The listing builds one solid part. Answer for the finished solid, in the listing's coordinates (mm). A direction names the side the tool comes from. Coordinates: 2 decimals unless noted, no trailing zeros. Write each loop counter-clockwise with the first axis right and the second up, starting at its lowest first coordinate (ties: lowest second). Pieces come first, ordered by that corner, then holes. Notation, with made-up numbers: M -21.5,36 L 12.5,36 A17 cw 12.5,46 Z; hole C 44,43.25 d1. An arc over 180 degrees is marked long. Answer as a JSON object with one key per item and string values. Group by question number.
Autodesk Inventor part; units mm, degrees
ref_plane "YZ Plane" through (0, 0, 0) normal (1, 0, 0) x (0, 1, 0)
ref_plane "XZ Plane" through (0, 0, 0) normal (0, 1, 0) x (-1, 0, 0)
ref_plane "XY Plane" through (0, 0, 0) normal (0, 0, 1) x (1, 0, 0)
sketch "Sketch1" plane through (0, 0, 0) normal (0, 0, 1) x (1, 0, 0)
  circle A0 centre (0, 0) radius 60.5
  circle A1 centre (0, 0) radius 55
  line L0 (0, 55) -> (-10, 55)
  line L1 (0, 55) -> (10, 55)
  line L2 (0, 55) -> (10, 55) construction
  line L3 (10, 59.6678) -> (10, 53.8845)
  line L4 (-10, 59.6678) -> (-10, 54.0833)
  point P0 (10, 54.0833)
  dimension "d0" = 121
  dimension "d1" = 110
  dimension "d45" = 10
  dimension "d46" = 10
  dimension "d47" = 0
extrude "Extrusion1" add sketch "Sketch1" along normal blind 2
extrude "Extrusion2" add sketch "Sketch1" against normal blind 8 contours A0 L4 A1 L3 | L3 L1 L0 L4 A0 | L3 A1 L1 | L0 A1 L4
sketch "Sketch11" plane through (0, 0, 0) normal (1, 0, 0) x (0, 1, 0)
  line L0 (60.5, 2) -> (-60.5, 2)
  line L1 (-60.5, -8) -> (60.5, -8)
  line L2 (59.6678, 0) -> (54.0833, 0)
  line L3 (59.6678, 0) -> (59.6678, -6)
  line L4 (54.0833, -6) -> (59.6678, -6)
  line L5 (54.0833, 0) -> (54.0833, -6)
  line L6 (-60.5, -8) -> (60.5, -8)
  line L7 (55, -8) -> (-55, -8)
  line L8 (-60.5, -8) -> (60.5, -8)
  line L9 (60.5, 0) -> (-60.5, 0)
  line L10 (-55, -8) -> (-61, -8)
  line L11 (-61, -8) -> (-61, 0)
  line L12 (-61, 0) -> (-55, 0)
  line L13 (-55, 0) -> (-55, -8)
  line L14 (-61, -8) -> (-55, 0)
  circle A0 centre (-58, -4) radius 2.1
  line L15 (-61, -8) -> (-67, -8)
  line L16 (-67, -8) -> (-67, -2)
  line L17 (-67, -2) -> (-61, -2)
  line L18 (-61, -2) -> (-61, -8)
  line L19 (-61, -8) -> (-67, -2)
  circle A1 centre (-64, -5) radius 2.15
  point P0 (0, 0)
  point P1 (42.0833, 0)
  point P2 (42.0833, -6)
  point P3 (48.0833, -6)
  dimension "d48" = 6
  dimension "d49" = 4.2
  dimension "d50" = 6
  dimension "d51" = 6
  dimension "d52" = 4.3
sketch "Sketch12" plane through (0, 0, 2) normal (0, 0, 1) x (1, 0, 0)
  point P0 (0, 0)
sketch "Sketch13" plane through (0, 0, 0) normal (0, 1, 0) x (-1, 0, 0)
  line L0 (0, -6) -> (0, 2)
  line L1 (0, 0) -> (0, -1)
  line L2 (0, -1) -> (3.1, -1)
  line L3 (3.1, -1) -> (3.1, -7.2)
  line L4 (3.1, -7.2) -> (0, -7.2)
  line L5 (0, -7.2) -> (0, -1)
  line L6 (3.1, -7.2) -> (-3.1, -7.2)
  line L7 (-3.1, -7.2) -> (-3.1, -1)
  line L8 (-3.1, -1) -> (3.1, -1)
  line L9 (3.1, -1) -> (3.1, -7.2)
  line L10 (0, -4.1) -> (6, -4.1)
  line L11 (6, -4.1) -> (-6, -4.1)
  circle A0 centre (-6, -4.1) radius 2.15
  circle A1 centre (6, -4.1) radius 2.15
  point P0 (0, -7.2)
  dimension "d58" = 1
  dimension "d59" = 3.1
  dimension "d60" = 6.2
  dimension "d61" = 6.2
  dimension "d62" = 6.2
  dimension "d66" = 6
  dimension "d67" = 12
  dimension "d68" = 4.3
  dimension "d69" = 4.3
extrude "Extrusion12" cut sketch "Sketch13" along normal through all
fillet "Fillet3" radius 0.3 4 edges at (-3.1, 57.6665, -1) (3.1, 57.6665, -1) (3.1, 57.6665, -7.2) (-3.1, 57.6665, -7.2)
sketch "Sketch14" plane through (0, 0, -8) normal (0, 0, -1) x (-1, 0, 0)
  circle A0 centre (0, 0) radius 57.5
  circle A1 centre (0, 57.5) radius 2.4
  circle A2 centre (-49.7965, -28.75) radius 2.4
  circle A3 centre (49.7965, -28.75) radius 2.4
  point P0 (50.9528, -26.6469)
  point P1 (48.5533, -30.803)
  dimension "d70" = 115
  dimension "d71" = 4.8
  dimension "d74" = 360
extrude "Extrusion13" add sketch "Sketch14" along normal blind 10 contours A1 A0 | A0 A1 | A0 A3 | A2 A0 | A0 A2 picked at (49.0578, -28.4334)
properties part number "Cover"
Item 1: A tool of negligible diameter and unlimited length cuts with its end or side. For faces 1 (the face through (50.317, -26.407, -12.93)), 2 (the face through (-13.12, 59.06, -3.07)), 3 (the face through (0, 58, -7.2)), from which of +Z, -Z, +X, -X, +Y, -Y can it reach the whole face along a straight path? Write none if from no direction.
Item 2: Consider L1, parallel to X at y = 0, z = -4.25; L2, parallel to Z at x = -6, y = 57.2; L3, parallel to Y at x = 0, z = -6. Determine where each line is inside the solid, lowest interval first. Write a range as from..to.
Item 3: Flat-ended cylindrical pins translate along their axes: pin 1 Ø6 at (y, z) = (58.5, -3) entering from +X; pin 2 Ø6 at (x, y) = (-11, 13.5) entering from -Z; pin 3 Ø4 at (x, z) = (-6, -4.1) entering from -Y; pin 4 Ø10 at (y, z) = (-3, -11.5) entering from -X. Find the tip coordinate at first contact, or state that the pin passes through.
Item 4: A cutting plane is placed at C-C, the plane y = 0. Write down the section's boundary in (x, z), and give its area (3 significant figures).
Item 5: A cutting plane is placed at B-B, the plane z = -4.1. Write down the section's boundary in (x, y).
Item 6: For a pull along X with two mould halves and no side action, classify faces 4 (the face through (-49.813, -28.721, -12.93)), 5 (the face through (-1, 1, 0)), 6 (the face through (-1.11, 59.63, -12.93)), 7 (the face through (-1, 1, 2)) as +X half, -X half, draft (parallel to the pull), parting line (faces both ways), or undercut.
Item 7: A cutting plane is placed at D-D, the plane y = 57.5. Write down the section's boundary in (x, z), and give its area (3 significant figures).
Item 8: A cutting plane is placed at A-A, the plane x = 0. Write down the section's boundary in (y, z).
Answer:
{
 "1": {"face 1": "-Z", "face 2": "+Z, -Z", "face 3": "+Y"},
 "2": {"L1": "-60.5..-55, 55..60.5", "L2": "-8..-6.25, -1.95..2", "L3": "-60.5..-55"},
 "3": {"pin 1": "x = 24.08", "pin 2": "z = 0", "pin 3": "y = -60.37", "pin 4": "x = -60.5"},
 "4": {"outline": "M -60.5,-8 L -55,-8 L -55,0 L 55,0 L 55,-8 L 60.5,-8 L 60.5,2 L -60.5,2 Z", "area": "330 mm2"},
 "5": {"outline": "M -8.15,54.39 L -8.15,59.95 A60.5 ccw long 8.15,59.95 L 8.15,54.39 A55 cw long Z; M -3.85,54.87 A55 cw -3.1,54.91 L -3.1,60.42 A60.5 ccw -3.85,60.38 Z; M 3.1,54.91 A55 cw 3.85,54.87 L 3.85,60.38 A60.5 ccw 3.1,60.42 Z"},
 "6": {"face 4": "-X half", "face 5": "undercut", "face 6": "parting line", "face 7": "draft"},
 "7": {"outline": "M -18.81,-8 L -2.4,-8 L -2.4,-18 L 2.4,-18 L 2.4,-8 L 18.81,-8 L 18.81,2 L -18.81,2 Z; hole C -6,-4.1 d4.3; hole M -3.1,-6.9 A0.3 ccw -2.8,-7.2 L 2.8,-7.2 A0.3 ccw 3.1,-6.9 L 3.1,-1.3 A0.3 ccw 2.8,-1 L -2.8,-1 A0.3 ccw -3.1,-1.3 Z; hole C 6,-4.1 d4.3", "area": "357 mm2"},
 "8": {"outline": "M -60.5,-8 L -55,-8 L -55,0 L 55,0 L 55,-1 L 60.5,-1 L 60.5,2 L -60.5,2 Z; M 55,-8 L 55.1,-8 L 55.1,-18 L 59.9,-18 L 59.9,-8 L 60.5,-8 L 60.5,-7.2 L 55,-7.2 Z"}
}
